Geometry check sheet. Reference: the model listing, model coordinates, mm. A direction names the side the tool comes from. Round coordinates to 2 decimals unless told otherwise and drop trailing zeros. Loops run counter-clockwise (first coordinate to the right, second up) from the corner with the lowest first, then second, coordinate; pieces in that order, holes last.
```python
from build123d import *

# Parameters (mm, degrees)
F4_W     = 3.175
F4_H     = 12.7
F5_DEPTH = 12.7


with BuildPart() as f2:
    # F0 (on Top) → F2 (revolve)
    with BuildSketch(Plane.XY):
        with BuildLine():
            Line((-35.4254181015, 31.2067266416), (-29.0754181015, 31.2067266416))
            Line((-29.0754181015, 31.2067266416), (-29.0754181015, 11.9027266416))
            Line((-29.0754181015, 11.9027266416), (-31.6154181015, 11.9027266416))
            Line((-31.6154181015, 11.9027266416), (-31.6154181015, 6.8227266416))
            Line((-31.6154181015, 6.8227266416), (-25.9004181015, 6.8227266416))
            Line((-25.9004181015, 6.8227266416), (-25.9004181015, 20.6251591444))
            Line((-25.9004181015, 20.6251591444), (-25.9004181015, 34.9045594707))
            add(Edge.make_bspline(
                [(-35.4254181015, 31.2067266416), (-32.3843405864, 32.9409682845), (-29.3432630713, 34.6752099275), (-25.9004181015, 34.9045594707)],
                knots=[0, 0, 0, 0, 0.3470016692, 0.3470016692, 0.3470016692, 0.3470016692], degree=3))
        make_face()
    revolve(axis=Axis((-25.7974471897, 17.4531694502, 0), (0, -1, 0)))

    # F4 (on face) → F5 (cut)
    with BuildSketch(Plane.XZ.offset(-6.8227266416)):
        with Locations((-25.7551228888, 0)):
            Rectangle(F4_W, F4_H)
    extrude(amount=-F5_DEPTH, mode=Mode.SUBTRACT)


solid = f2.part
```
1) Gauge pin test, flat ends, axial feed: pin 1 (1 mm diameter, centred on y = 32, z = 3, fed in from +X); pin 2 (10 mm diameter, centred on y = 22.5, z = -1.5, fed in from -X); pin 3 (1.3 mm diameter, centred on x = -30.5, z = 1, fed in from +Y). Record the tip position at first contact, or that the pin passes through.
Report:
pin 1: stops at x = -17.18
pin 2: stops at x = -29.08
pin 3: stops at y = 33.97
2) Sectioned sample at A-A, the plane y = 30.75. Record the cut outline in (x, z), then the cut area to 3 significant figures.
Report:
outline: circle Ø6.56 at (-25.8, 0); hole circle Ø0.21 at (-25.8, 0)
area: 33.7 mm2
3) Mould release check, pull along X, two halves, no side actions. Record for faces 1 (the face through (-27.343, 12, 0)), 2 (the face through (-19.98, 9.33, -0.1)), 3 (the face through (-29, 6.823, 0)), 4 (the face through (-31.614, 9.327, 0.106)): +X half, -X half, draft (parallel to the pull), parting line (faces both ways), or undercut.
Report:
face 1: undercut
face 2: +X half
face 3: draft
face 4: -X half
4) Scan lines: line 1 along X through (y, z) = (23.25, 0); line 2 along Y through (x, z) = (-21, -2); line 3 along X through (y, z) = (10, 1.25). Record each from-to range of solid material in increasing order.
Report:
line 1: x = -29.08 to -25.9, -25.69 to -22.52
line 2: y = 6.82 to 11.9, 31.21 to 33.54
line 3: x = -31.48 to -27.34, -24.17 to -20.12
5) Sectioned sample at B-B, the plane z = -5. State how many separate pieces and enclosed holes the cut face has, then the cut area to 4 significant figures.
Report:
separate pieces: 3
enclosed holes: 0
area: 39.65 mm2
6) Sectioned sample at C-C, the plane y = 16.25. Record the cut outline in (x, z), then the cut area to 3 significant figures.
Report:
outline: (-27.34, -2.89) - (-27.34, 2.89) arc R3.28 ccw to start; (-24.17, -2.84) arc R3.28 ccw to (-24.17, 2.84) - close
area: 13.8 mm2
7) Access from +Z, -Z, +X, -X, +Y, -Y to the whole of each face (thin tool, end or side, straight path). Record for faces 5 (the face through (-26.1, 19.523, 0)), 6 (the face through (-30, 11.903, 0)), 7 (the face through (-22, 11.903, 0)), 8 (the face through (-25.37, 21.42, -3.25)).
Report:
face 5: +Z, -Z, -Y
face 6: -X
face 7: +X
face 8: none
